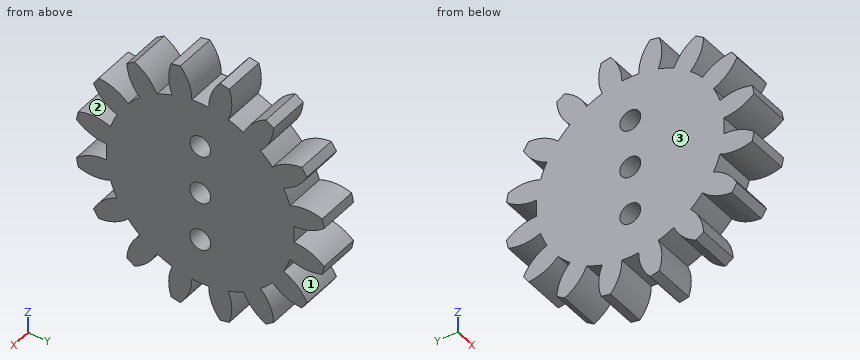
```python
from build123d import *

# Parameters (mm, degrees)
BASPROSKE_W             = 6
BASPROSKE_H             = 18
TOOTHCUT_DEPTH          = 27.153393661
TEETHCUTS_COUNT         = 16
TEETHCUTS_ANGLE         = 337.5
BORSKE_R                = 4
BORE_DEPTH              = 50.0000508
CROQUIS1_R              = 4
CROQUIS1_R_2            = 1.5
SALIENTE_EXTRUIR1_DEPTH = 6
CROQUIS2_R              = 1.5
CORTAR_EXTRUIR1_DEPTH   = 6


with BuildPart() as part:
    # BasProSke → Base-Revolve (revolve)
    with BuildSketch(Plane(origin=(0, 0, 0), x_dir=(1, 0, 0), z_dir=(0, 1, 0)), mode=Mode.PRIVATE) as base_revolve_sk:
        with Locations((3, 9)):
            Rectangle(BASPROSKE_W, BASPROSKE_H)
    revolve(base_revolve_sk.sketch.rotate(Axis((-10, 0, 0), (1, 0, 0)), 180), axis=Axis((-10, 0, 0), (1, 0, 0)))

    # TooCutSke → ToothCut (cut, through all)
    with BuildSketch(Plane(origin=(0, 0, 0), x_dir=(0, 0, -1), z_dir=(1, 0, 0))):
        with BuildLine():
            ThreePointArc((1.210794474, 13.444589162), (0, 13.499), (-1.210794474, 13.444589162))
            ThreePointArc((-1.210794474, 13.444589162), (-1.632237109, 15.776340848), (-2.873179402, 17.794939879))
            ThreePointArc((-2.873179402, 17.794939879), (0, 18.0254), (2.873179402, 17.794939879))
            ThreePointArc((2.873179402, 17.794939879), (1.632237109, 15.776340848), (1.210794474, 13.444589162))
        make_face()
    toothcut = extrude(amount=TOOTHCUT_DEPTH, mode=Mode.SUBTRACT)

    # TeethCuts: ToothCut ×16 about axis
    teethcuts_axis = Axis((-10, 0, 0), (1, 0, 0))
    for i in range(1, TEETHCUTS_COUNT):
        add(toothcut.rotate(teethcuts_axis, i * TEETHCUTS_ANGLE / (TEETHCUTS_COUNT - 1)), mode=Mode.SUBTRACT)

    # BorSke → Bore (cut, symmetric)
    with BuildSketch(Plane(origin=(0, 0, 0), x_dir=(0, 0, -1), z_dir=(1, 0, 0))):
        with Locations(Location((0, 0, 0), (0, 0, 180))):
            Circle(BORSKE_R)
    extrude(amount=BORE_DEPTH, both=True, mode=Mode.SUBTRACT)

    # Croquis1 → Saliente-Extruir1 (add)
    with BuildSketch(Plane(origin=(6, 0, 0), x_dir=(0, 0, -1), z_dir=(1, 0, 0))):
        Circle(CROQUIS1_R)
        Circle(CROQUIS1_R_2, mode=Mode.SUBTRACT)
    extrude(amount=-SALIENTE_EXTRUIR1_DEPTH)

    # Croquis2 → Cortar-Extruir1 (cut)
    with BuildSketch(Plane(origin=(6, 0, 0), x_dir=(0, 0, -1), z_dir=(1, 0, 0))):
        with Locations((-7, 0)):
            Circle(CROQUIS2_R)
        with Locations((7, 0)):
            Circle(CROQUIS2_R)
    extrude(amount=-CORTAR_EXTRUIR1_DEPTH, mode=Mode.SUBTRACT)


solid = part.part
```
Can you work these out from the model? Positions are in its coordinate system, mm. Face numbers are marked on the shaded views. Give positions to 0.01 mm unless a question says otherwise; leave off trailing zeros. Write each loop counter-clockwise with the first axis right and the second up, starting at its lowest first coordinate (ties: lowest second). Pieces come first, ordered by that corner, then holes. Notation, with made-up numbers: (-5, 19.5) -> (53, 19.5) arc R31 cw to (53, 45.5) -> close; hole circle Ø6 at (1, 7). An arc over 180 degrees is marked (long way). One line per item, written item: value.
Q1. Imagine slicing it at A-A on z = 0. Please give me the cut outline in (x, y).
Results found:
outline: (0, -13.5) -> (6, -13.5) -> (6, -1.5) -> (0, -1.5) -> close; (0, 1.5) -> (6, 1.5) -> (6, 13.5) -> (0, 13.5) -> close
Q2. Please list where these lines run through material, in increasing order: line 1 (Z direction, x = 1.05, y = 9.5); line 2 (Y direction, x = 1.1, z = -9); line 3 (Y direction, x = 2.4, z = 6). Write a range as [from, to].
Results found:
line 1: z = [-15.29, -11.4], [-9.59, 9.59], [11.4, 15.29]
line 2: y = [-15.1, -10.74], [-10.06, 10.06], [10.74, 15.1]
line 3: y = [-12.09, -1.12], [1.12, 12.09]
Q3. Imagine slicing it at D-D on y = 11.5. Please give me the cut outline in (x, z).
Results found:
outline: (0, -9.57) -> (6, -9.57) -> (6, 9.57) -> (0, 9.57) -> close
Q4. We'd pull the mould along Y, two halves only. Please class the marked faces 1, 2 and 3: +Y half, -Y half, draft (parallel to the pull), parting line (faces both ways), or undercut.
Results found:
face 1: +Y half
face 2: undercut
face 3: draft
Q5. For P1, Ø1, axis at x = 1.5, y = -14, coming from the +Z side; P2, Ø1.5, axis at x = 0.5, z = 10, coming from the -Y side, each with a flat end and sliding along its axis, tell me the tip position at first contact or that it passes through.
Results found:
P1: stops at z = 10.54
P2: stops at y = -15.33
Q6. Imagine slicing it at B-B on x = 1.65. Give the number of separate pieces and of enclosed holes in the cut face, and give its area (3 significant figures).
Results found:
separate pieces: 1
enclosed holes: 3
area: 746 mm^2
Q7. Imagine slicing it at C-C on z = -7. Please give me the cut outline in (x, y), and give its area (3 significant figures).
Results found:
outline: (0, -13.29) -> (6, -13.29) -> (6, -1.5) -> (0, -1.5) -> close; (0, 1.5) -> (6, 1.5) -> (6, 13.29) -> (0, 13.29) -> close
area: 141 mm^2
